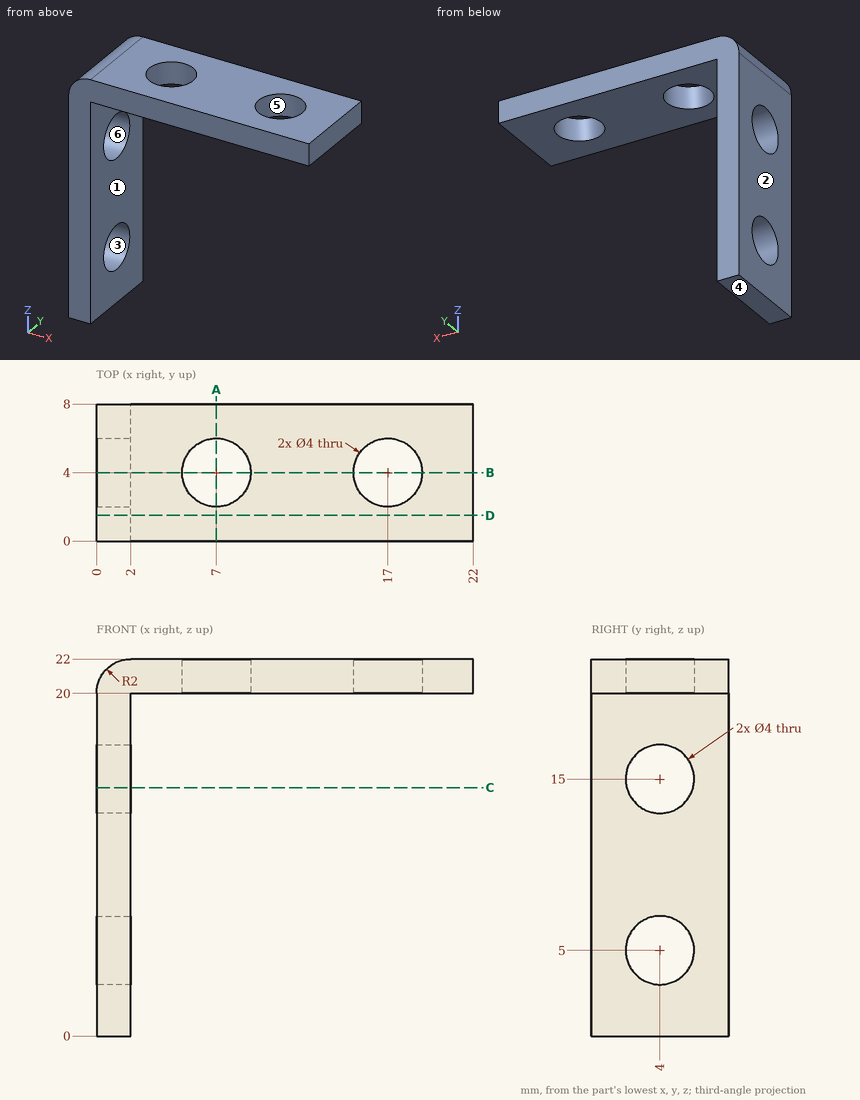
Print and shaded views of the part. All mm, measured from the part's lowest x, y and z. A direction names the side the tool comes from. Round coordinates to 2 decimals unless told otherwise and drop trailing zeros. Write each loop counter-clockwise with the first axis right and the second up, starting at its lowest first coordinate (ties: lowest second). Pieces come first, ordered by that corner, then holes. Notation, with made-up numbers: (42.25, 57) -> (83.25, 57) arc R7 cw to (83.25, 64) -> close; hole circle Ø5 at (49.25, 30.25). An arc over 180 degrees is marked (long way). Return JSON: item names as keys, results as strings. Group by question number.
Q1. Mould opens along Z. For the marked faces 3, 4, 5 and 6 say: pulls with the +Z half, pulls with the -Z half, needs draft (parallel to the pull), parting line crosses it, or undercut.
Q2. Saw through at C-C on z = 14.5. Write the cut outline in (x, y), plus the area to 3 significant figures.
Q3. Saw through at B-B on y = 4. Write the cut outline in (x, z).
Q4. Saw through at A-A on x = 7. Write the cut outline in (y, z), plus the area to 3 significant figures.
Q5. Probe L1, parallel to Y at x = 17, z = 20.4; L2, parallel to X at y = 3, z = 21.25; L3, parallel to X at y = 7.25, z = 4.75. List the from-to ranges inside material, lowest first. Write a range as [from, to].
Q6. Pin check, flat tips, straight feed: pin 1 (3.5 mm diameter, centred on y = 4, z = 15, fed in from -X); pin 2 (2 mm diameter, centred on y = 5, z = 15.5, fed in from +X); pin 3 (2.5 mm diameter, centred on x = 12, y = 5, fed in from -Z). Stop position of each tip, or through.
Q7. Saw through at D-D on y = 1.5. Write the cut outline in (x, z).
Q8. Which spindle directions (+Z, -Z, +X, -X, +Y, -Y) get a long thin tool onto all of the face, cutting with end or side? Do the marked faces 1 and 2. Say none if no direction does.
Answer:
{
 "1": {"face 3": "undercut", "face 4": "pulls with the -Z half", "face 5": "needs draft", "face 6": "undercut"},
 "2": {"outline": "(0, 0) -> (2, 0) -> (2, 2.06) -> (0, 2.06) -> close; (0, 5.94) -> (2, 5.94) -> (2, 8) -> (0, 8) -> close", "area": "8.25 mm2"},
 "3": {"outline": "(0, 0) -> (2, 0) -> (2, 3) -> (0, 3) -> close; (0, 7) -> (2, 7) -> (2, 13) -> (0, 13) -> close; (0, 17) -> (2, 17) -> (2, 20) -> (5, 20) -> (5, 22) -> (2, 22) arc R2 ccw to (0, 20) -> close; (9, 20) -> (15, 20) -> (15, 22) -> (9, 22) -> close; (19, 20) -> (22, 20) -> (22, 22) -> (19, 22) -> close"},
 "4": {"outline": "(0, 20) -> (2, 20) -> (2, 22) -> (0, 22) -> close; (6, 20) -> (8, 20) -> (8, 22) -> (6, 22) -> close", "area": "8.00 mm2"},
 "5": {"L1": "[0, 2], [6, 8]", "L2": "[0.44, 5.27], [8.73, 15.27], [18.73, 22]", "L3": "[0, 2]"},
 "6": {"pin 1": "through", "pin 2": "x = 2", "pin 3": "z = 20"},
 "7": {"outline": "(0, 0) -> (2, 0) -> (2, 20) -> (22, 20) -> (22, 22) -> (2, 22) arc R2 ccw to (0, 20) -> close"},
 "8": {"face 1": "-Z, +X, +Y, -Y", "face 2": "+Z, -Z, -X, +Y, -Y"}
}
